Source: CAD feature listing. Evaluate the final solid. Frame: model axes, mm. Face numbers are marked on the shaded views. A direction names the side the tool comes from. Coordinates: 2 decimals unless noted, no trailing zeros. Write each loop counter-clockwise with the first axis right and the second up, starting at its lowest first coordinate (ties: lowest second). Pieces come first, ordered by that corner, then holes. Notation, with made-up numbers: M 50,38.25 L 88,38.25 A11 cw 88,55.25 Z; hole C 19,-31 d7. An arc over 180 degrees is marked long. Write item = value, one per line. Start each with the question number.
1. Section query D-D (x = -1.75). Output: boundary loops of the cut face in (y, z).
2. Section query C-C (z = 5.25). Output: boundary loops of the cut face in (x, y).
3. Section query B-B (y = -1.25). Output: boundary loops of the cut face in (x, z).
4. Pull-direction query (X, two-part tool) for the marked faces 1, 2 and 3; classes: pulls with the +X half, pulls with the -X half, needs draft (parallel to the pull), parting line crosses it, or undercut.
5. Section query A-A (z = 1). Output: boundary loops of the cut face in (x, y).
6. Access query for the marked faces 4 and 5. Directions: +Z, -Z, +X, -X, +Y, -Y. A direction counts if a zero-diameter tool reaches every point of the face in a straight line with its end or side. Return the directions, or none.
7. Pin query (flat end, axial travel): pin 1 Ø1.5 at (x, y) = (-1, 0.5) entering from +Z; pin 2 Ø1.5 at (x, y) = (5, 1) entering from -Z; pin 3 Ø1.5 at (x, y) = (-2.5, 0) entering from -Z. Return the tip coordinate at first contact, or that it passes through.
8. Line query: line 1 along X through (y, z) = (-0.3, 1.25); line 2 along X through (y, z) = (1.45, 6.5); line 3 along Z through (x, y) = (-3.25, -0.45). Output: solid intervals per line, ascending.
```python
from build123d import *

# Parameters (mm, degrees)
BOSS_EXTRUDE1_DEPTH = 1.5


with BuildPart() as part:
    # Sketch1 → Boss-Extrude1 (new, symmetric)
    with BuildSketch(Plane(origin=(0, 0, 0), x_dir=(1, 0, 0), z_dir=(0, 1, 0))):
        with BuildLine():
            Line((-7.5, -2.783882181), (-7.5, 0.216117819))
            Line((-7.5, 0.216117819), (-6.646806682, 0.216117819))
            Line((-6.646806682, 0.216117819), (-6.646806682, -2.783882181))
            ThreePointArc((-6.646806682, -2.783882181), (0, -7.20625), (6.646806682, -2.783882181))
            Line((6.646806682, -2.783882181), (6.646806682, 0.216117819))
            Line((6.646806682, 0.216117819), (7.5, 0.216117819))
            Line((7.5, 0.216117819), (7.5, -2.783882181))
            ThreePointArc((7.5, -2.783882181), (0, -8), (-7.5, -2.783882181))
        make_face()
    extrude(amount=BOSS_EXTRUDE1_DEPTH, both=True)


solid = part.part
```
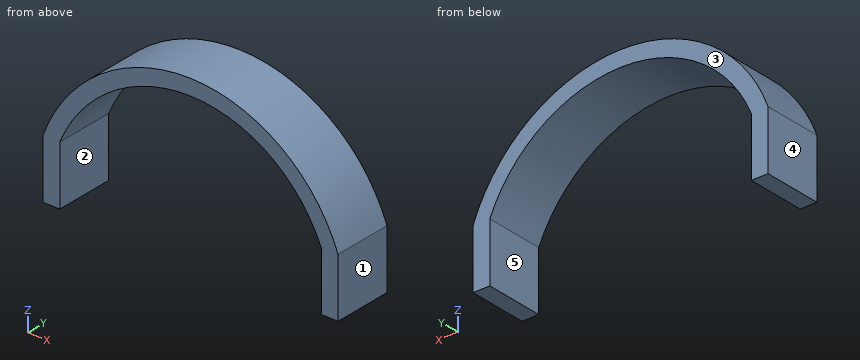
Results are:
q1.outline = M -1.5,6.99 L 1.5,6.99 L 1.5,7.81 L -1.5,7.81 Z
q2.outline = M -6.04,-1.5 L -4.94,-1.5 L -4.94,1.5 L -6.04,1.5 Z; M 4.94,-1.5 L 6.04,-1.5 L 6.04,1.5 L 4.94,1.5 Z
q3.outline = M -7.5,-0.22 L -6.65,-0.22 L -6.65,2.78 A7.21 cw 6.65,2.78 L 6.65,-0.22 L 7.5,-0.22 L 7.5,2.78 A8 ccw -7.5,2.78 Z
q4.face_1 = pulls with the +X half
q4.face_2 = undercut
q4.face_3 = needs draft
q5.outline = M -7.5,-1.5 L -6.65,-1.5 L -6.65,1.5 L -7.5,1.5 Z; M 6.65,-1.5 L 7.5,-1.5 L 7.5,1.5 L 6.65,1.5 Z
q6.face_4 = +Z, -Z, -X, +Y, -Y
q6.face_5 = -Z, +Y, -Y
q7.pin_1 = 8
q7.pin_2 = 4.34
q7.pin_3 = 6.43
q8.line_1 = -7.5 to -6.65, 6.65 to 7.5
q8.line_2 = -4.66 to -3.11, 3.11 to 4.66
q8.line_3 = 6.43 to 7.31
